from build123d import *
from build123d.topology import SkipClean

# Parameters (mm, degrees)
BOSS_EXTRUDE2_DEPTH = 4
SKETCH4_R           = 2.5
CUT_EXTRUDE1_DEPTH  = 19.788294228
SKETCH6_R           = 12.5
BOSS_EXTRUDE3_DEPTH = 4
BOSS_EXTRUDE4_DEPTH = 1.5
BOSS_EXTRUDE5_DEPTH = 10
CUT_EXTRUDE2_REACH  = 44.364
SKETCH9_W           = 1
SKETCH9_H           = 7


with BuildPart() as part:
    # Sketch3 → Boss-Extrude2 (new, symmetric)
    with BuildSketch(Plane.XY):
        with BuildLine():
            Line((8, 0), (8, -15))
            Line((8, -15), (-8, -15))
            Line((-8, -15), (-8, 0))
            ThreePointArc((-8, 0), (0, 8), (8, 0))
        make_face()
    extrude(amount=BOSS_EXTRUDE2_DEPTH, both=True)

    # Sketch4 → Cut-Extrude1 (cut, through all)
    with BuildSketch(Plane(origin=(0, 0, -4), x_dir=(-1, 0, 0), z_dir=(0, 0, -1))):
        Circle(SKETCH4_R)
    extrude(amount=-CUT_EXTRUDE1_DEPTH, mode=Mode.SUBTRACT)

    # Sketch6 → Boss-Extrude3 (add)
    with BuildSketch(Plane.XZ.offset(15)):
        with Locations(Location((0, 0, 0), (0, 0, 270))):
            Circle(SKETCH6_R)
    extrude(amount=BOSS_EXTRUDE3_DEPTH)

    # Sketch7 → Boss-Extrude4 (add)
    with SkipClean():  # the faces are left unmerged after this step: merging them gives an invalid solid
        with BuildSketch(Plane.XZ.offset(19)):
            with BuildLine():
                Line((-12.5, 0), (-10.5, 0))
                ThreePointArc((-10.5, 0), (0, -10.5), (10.5, 0))
                Line((10.5, 0), (12.5, 0))
                ThreePointArc((12.5, 0), (0, -12.5), (-12.5, 0))
            make_face()
        extrude(amount=BOSS_EXTRUDE4_DEPTH)
    add(part.part.scale(1), mode=Mode.REPLACE)  # the faces are merged on a copy

    # Sketch8 → Boss-Extrude5 (add)
    with SkipClean():  # the faces are left unmerged after this step: merging them gives an invalid solid
        with BuildSketch(Plane.XZ.offset(20.5)):
            with BuildLine():
                Line((-12.5, 0), (12.5, 0))
                ThreePointArc((12.5, 0), (0, -12.5), (-12.5, 0))
            make_face()
        extrude(amount=BOSS_EXTRUDE5_DEPTH)

    # Sketch9 → Cut-Extrude2 (cut, up to next)
    with BuildSketch(Plane.XZ.offset(30.5), mode=Mode.PRIVATE) as cut_extrude2_sk1:
        with Locations((0, -3.5)):
            Rectangle(SKETCH9_W, SKETCH9_H)
    cut_extrude2_tool1 = extrude(cut_extrude2_sk1.sketch, amount=-CUT_EXTRUDE2_REACH, mode=Mode.PRIVATE) & part.part
    add(cut_extrude2_tool1.solids().sort_by_distance((0, -30.5, -3.5))[0], mode=Mode.SUBTRACT)


solid = part.part
Check sheet for the modelled part. Datum: model origin and axes. Units: mm. A direction names the side the tool comes from. Round coordinates to 2 decimals unless told otherwise and drop trailing zeros. Loops run counter-clockwise (first coordinate to the right, second up) from the corner with the lowest first, then second, coordinate; pieces in that order, holes last.
1. Mould release check, pull along X, two halves, no side actions. Record for faces 6 (the flat face through (-8, -8, 0)), 7 (the flat face through (2, -20.5, -4)), 8 (the flat face through (0.5, -26, -4)), 9 (the flat face through (-7, -25, 0)): released by +X, released by -X, zero draft, split by the parting line, or undercut.
2. Gauge pin test, flat ends, axial feed: pin 1 Ø9 at (y, z) = (-10, -1) entering from +X; pin 2 Ø9 at (x, y) = (-4, -26.5) entering from +Z; pin 3 Ø5.5 at (y, z) = (-23, -4) entering from +X; pin 4 Ø11.5 at (x, z) = (2, -4) entering from +Y. Record the tip position at first contact, or that the pin passes through.
3. Sectioned sample at A-A on x = 0. Record the boundary of the cut face in (y, z).
4. Scan lines: probe 1 along Y at (x, z) = (0, -1.5); probe 2 along X at (y, z) = (-23, -2); probe 3 along Y at (x, z) = (3, 8.5). Record each from-to range of solid material in increasing order.
5. Sectioned sample at B-B on z = -1.25. Record the boundary of the cut face in (x, y).
6. Sectioned sample at C-C on y = -15.5. Record the boundary of the cut face in (x, z), and give its area (3 significant figures).
7. Sectioned sample at D-D on x = -6. Record the boundary of the cut face in (y, z), and give its area (3 significant figures).
8. Set-up check for faces 1 (the flat face through (8, -7, 0)), 2 (the cylindrical face through (-0.2, -19.7, -10.5)), 3 (the flat face through (0, -3, 4)), 4 (the flat face through (0, -26, -7)), 5 (the flat face through (0, -3, -4)): record each of +Z, -Z, +X, -X, +Y, -Y from which the full face is reachable in a straight line by a thin tool's end or side.
Recorded:
1. face 6: released by -X
1. face 7: undercut
1. face 8: undercut
1. face 9: zero draft
2. pin 1: stops at x = 8
2. pin 2: stops at z = 0
2. pin 3: stops at x = 12.44
2. pin 4: stops at y = 8
3. outline: (-30.5, -12.5) - (-15, -12.5) - (-15, -4) - (-2.5, -4) - (-2.5, 4) - (-15, 4) - (-15, 12.5) - (-19, 12.5) - (-19, -10.5) - (-20.5, -10.5) - (-20.5, -7) - (-30.5, -7) - close; (2.5, -4) - (8, -4) - (8, 4) - (2.5, 4) - close
4. probe 1: y = -19 to -2.5, 2.5 to 8
4. probe 2: x = -12.34 to -0.5, 0.5 to 12.34
4. probe 3: y = -19 to -15
5. outline: (-12.44, -30.5) - (-0.5, -30.5) - (-0.5, -20.5) - (-10.43, -20.5) - (-10.43, -19) - (10.43, -19) - (10.43, -20.5) - (0.5, -20.5) - (0.5, -30.5) - (12.44, -30.5) - (12.44, -15) - (8, -15) - (8, 0) arc R8 ccw to (-8, 0) - (-8, -15) - (-12.44, -15) - close; hole circle Ø5 at (0, 0)
6. outline: circle Ø25 at (0, 0)
6. area: 491 mm2
7. outline: (-30.5, -10.97) - (-15, -10.97) - (-15, -4) - (5.29, -4) - (5.29, 4) - (-15, 4) - (-15, 10.97) - (-19, 10.97) - (-19, -8.62) - (-20.5, -8.62) - (-20.5, 0) - (-30.5, 0) - close
7. area: 363 mm2
8. face 1: +Z, -Z, +X, +Y
8. face 2: +Z
8. face 3: +Z, +X, -X, +Y
8. face 4: +Z, -Y
8. face 5: -Z, +X, -X, +Y
